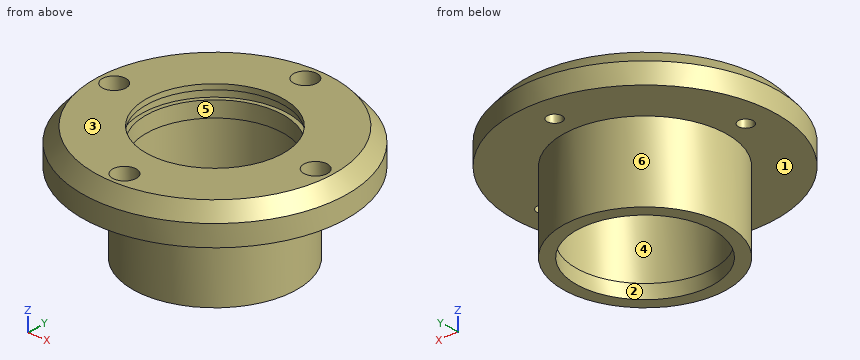
from build123d import *

# Parameters (mm, degrees)
F4_R     = 4.25
F5_DEPTH = 25
F4_R_2   = 6.75
F6_DEPTH = 8
F7_DEPTH = 8
F8_DEPTH = 8


with BuildPart() as f1:
    # F0 (on Front) → F1 (revolve)
    with BuildSketch(Plane.XZ):
        Polygon((75, 57), (68, 65), (39, 65), (39, 62), (41.5, 62), (41.5, 57), (39, 57), (39, 48), (40.5, 48), (40.5, 8), (39, 8), (39, 0), (46.5, 0), (46.5, 45), (75, 45), align=None)
    revolve(axis=Axis((0, 0, 14.0173053369), (0, 0, -1)))

    # F4 (on offset) → F5 (cut)
    with BuildSketch(Plane.XY.offset(65)):
        with Locations((0, 59)):
            Circle(F4_R)
        with Locations((-59, 0)):
            Circle(F4_R)
        with Locations((0, -59)):
            Circle(F4_R)
        with Locations((59, 0)):
            Circle(F4_R)
    extrude(amount=-F5_DEPTH, mode=Mode.SUBTRACT)

    # F4 (on offset) → F6 (cut)
    with BuildSketch(Plane.XY.offset(65)):
        with Locations((0, 59)):
            Circle(F4_R_2)
        with Locations((0, 59)):
            Circle(F4_R, mode=Mode.SUBTRACT)
    extrude(amount=-F6_DEPTH, mode=Mode.SUBTRACT)

    # F4 (on offset) → F7 (cut)
    with BuildSketch(Plane.XY.offset(65)):
        with Locations((-59, 0)):
            Circle(F4_R_2)
        with Locations((-59, 0)):
            Circle(F4_R, mode=Mode.SUBTRACT)
        with Locations((59, 0)):
            Circle(F4_R_2)
        with Locations((59, 0)):
            Circle(F4_R, mode=Mode.SUBTRACT)
        with Locations((0, -59)):
            Circle(F4_R_2)
        with Locations((0, -59)):
            Circle(F4_R, mode=Mode.SUBTRACT)
    extrude(amount=-F7_DEPTH, mode=Mode.SUBTRACT)

    # F4 (on offset) → F8 (cut)
    with BuildSketch(Plane.XY.offset(65)):
        with Locations((0, -59)):
            Circle(F4_R_2)
        with Locations((0, -59)):
            Circle(F4_R, mode=Mode.SUBTRACT)
    extrude(amount=-F8_DEPTH, mode=Mode.SUBTRACT)


solid = f1.part
The model under review builds one solid part; all positions refer to its coordinate system, in mm. Face numbers are marked on the shaded views. A direction names the side the tool comes from. Give positions to 0.01 mm unless a question says otherwise; leave off trailing zeros. Write each loop counter-clockwise with the first axis right and the second up, starting at its lowest first coordinate (ties: lowest second). Pieces come first, ordered by that corner, then holes.
1. Add section A-A, the plane z = 41.5. Write out the cut boundary in (x, y).
2. Add section B-B, the plane y = 0. Count the separate pieces of the cut face and the enclosed holes in it, plus the area to 3 significant figures.
3. Wall thickness on L1, parallel to Y at x = 0, z = 50; L2, parallel to Y at x = 0, z = 33: over which ranges is each line inside the solid? List them lowest first.
4. Draft analysis for pull direction X (two halves, no side actions). For the marked faces 3, 4, 5 and 6, state which applies: +X half, -X half, draft (parallel to the pull), parting line (faces both ways), or undercut.
5. Tool access review of the marked faces 1 and 2: name each direction out of +Z, -Z, +X, -X, +Y, -Y from which nothing blocks a thin tool from reaching the whole face with its end or side.
6. For P1, Ø6, axis at x = -28, z = 44, coming from the -Y side; P2, Ø7, axis at x = 59, y = 0, coming from the -Z side; P3, Ø7, axis at x = -61, y = 2, coming from the +Z side; P4, Ø2, axis at y = 23, z = 8.5, coming from the -X side, all flat-tipped, find the tip position at first contact; note any pin that passes through.
Worked answers:
1. outline: circle Ø93 at (0, 0); hole circle Ø81 at (0, 0)
2. separate pieces: 4
2. enclosed holes: 0
2. area: 1,490 mm2
3. L1: y = -75 to -63.25, -54.75 to -39, 39 to 54.75, 63.25 to 75
3. L2: y = -46.5 to -40.5, 40.5 to 46.5
4. face 3: draft
4. face 4: undercut
4. face 5: undercut
4. face 6: parting line
5. face 1: -Z
5. face 2: +Z, -Z
6. P1: stops at y = -70.65
6. P2: passes through
6. P3: stops at z = 57
6. P4: stops at x = -40.97
